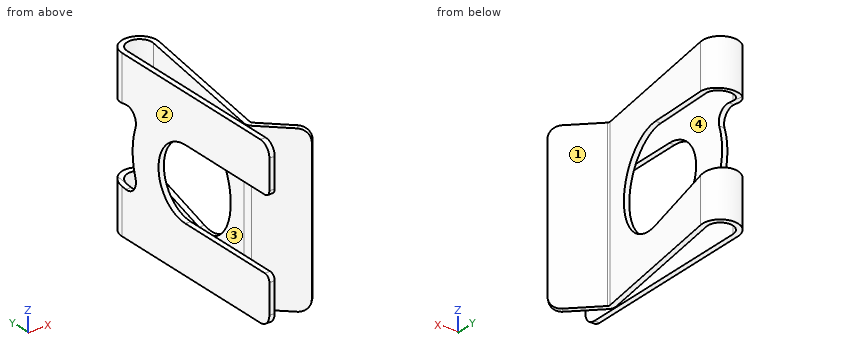
```python
from build123d import *

# Parameters (mm, degrees)
BOSS_EXTRUDE1_DEPTH      = 7
BOSS_EXTRUDE1_DEPTH_BACK = 7
CUT_EXTRUDE1_DEPTH       = 0.45
CUT_EXTRUDE2_DEPTH       = 3.9
CUT_EXTRUDE3_DEPTH       = 3.9
CUT_EXTRUDE4_DEPTH       = 0.45
CUT_EXTRUDE5_DEPTH       = 0.45
CUT_EXTRUDE6_DEPTH       = 0.45
CUT_EXTRUDE7_DEPTH       = 0.45
CUT_EXTRUDE8_DEPTH       = 0.9
CUT_EXTRUDE8_DEPTH_BACK  = 0.9


with BuildPart() as part:
    # Sketch1 → Boss-Extrude1 (new body, two sides)
    with BuildSketch(Plane.XY) as boss_extrude1_sk:
        with BuildLine():
            Line((0, 7.1), (0, -9.4))
            Line((0, -9.4), (0.45, -9.4))
            Line((0.45, -9.4), (0.45, 7.1))
            ThreePointArc((0.45, 7.1), (1.582064395, 8.146788152), (2.537172257, 6.936373264))
            Line((2.537172257, 6.936373264), (0.513952578, -5.888103783))
            ThreePointArc((0.513952578, -5.888103783), (0.540554577, -6.207374008), (0.711367038, -6.478416895))
            Line((0.711367038, -6.478416895), (3.64329211, -9.314940681))
            Line((3.64329211, -9.314940681), (3.956184866, -8.99152435))
            Line((3.956184866, -8.99152435), (1.024259794, -6.155000564))
            ThreePointArc((1.024259794, -6.155000564), (0.967322307, -6.064652935), (0.958454974, -5.958229527))
            Line((0.958454974, -5.958229527), (2.981674653, 6.86624752))
            ThreePointArc((2.981674653, 6.86624752), (1.61723485, 8.595411646), (0, 7.1))
        make_face()
    extrude(amount=BOSS_EXTRUDE1_DEPTH)
    extrude(boss_extrude1_sk.sketch, amount=-BOSS_EXTRUDE1_DEPTH_BACK)

    # Sketch2 → Cut-Extrude1 (cut)
    with BuildSketch(Plane(origin=(0, 0, 0), x_dir=(0, 0, -1), z_dir=(1, 0, 0))):
        with BuildLine():
            Line((-3, 0), (-3, -9.4))
            Line((-3, -9.4), (3, -9.4))
            Line((3, -9.4), (3, 0))
            ThreePointArc((3, 0), (0, 3), (-3, 0))
        make_face()
    extrude(amount=CUT_EXTRUDE1_DEPTH, mode=Mode.SUBTRACT)

    # Sketch3 → Cut-Extrude2 (cut)
    with BuildSketch(Plane(origin=(0.45, 0, 0), x_dir=(0, 0, -1), z_dir=(1, 0, 0))):
        with BuildLine():
            Line((3.97169805, 0.474989052), (3, 8.6))
            Line((3, 8.6), (-3, 8.6))
            Line((-3, 8.6), (-3.97169805, 0.474989052))
            ThreePointArc((-3.97169805, 0.474989052), (0, -4), (3.97169805, 0.474989052))
        make_face()
    extrude(amount=CUT_EXTRUDE2_DEPTH, mode=Mode.SUBTRACT)

    # Sketch4 → Cut-Extrude3 (cut)
    with BuildSketch(Plane(origin=(0.45, 0, 0), x_dir=(0, 0, -1), z_dir=(1, 0, 0))):
        with BuildLine():
            Line((3.233838828, 6.644718687), (3, 8.6))
            Line((3, 8.6), (-3, 8.6))
            Line((-3, 8.6), (-3.233838828, 6.644718687))
            ThreePointArc((-3.233838828, 6.644718687), (-2.869340143, 5.748101911), (-1.916144125, 5.580178464))
            ThreePointArc((-1.916144125, 5.580178464), (0, 5.9), (1.916144125, 5.580178464))
            ThreePointArc((1.916144125, 5.580178464), (2.869340143, 5.748101911), (3.233838828, 6.644718687))
        make_face()
    extrude(amount=-CUT_EXTRUDE3_DEPTH, mode=Mode.SUBTRACT)

    # Sketch5 → Cut-Extrude4 (cut)
    with BuildSketch(Plane(origin=(0, 0, 0), x_dir=(0, 0, -1), z_dir=(1, 0, 0))):
        with BuildLine():
            Line((-7, -9.4), (-6, -9.4))
            ThreePointArc((-6, -9.4), (-6.707106781, -9.107106781), (-7, -8.4))
            Line((-7, -8.4), (-7, -9.4))
        make_face()
    extrude(amount=CUT_EXTRUDE4_DEPTH, mode=Mode.SUBTRACT)

    # Sketch6 → Cut-Extrude5 (cut)
    with BuildSketch(Plane(origin=(0, 0, 0), x_dir=(0, 0, -1), z_dir=(1, 0, 0))):
        with BuildLine():
            Line((6, -9.4), (7, -9.4))
            Line((7, -9.4), (7, -8.4))
            ThreePointArc((7, -8.4), (6.707106781, -9.107106781), (6, -9.4))
        make_face()
    extrude(amount=CUT_EXTRUDE5_DEPTH, mode=Mode.SUBTRACT)

    # Sketch7 → Cut-Extrude6 (cut)
    with BuildSketch(Plane(origin=(0, 0, 0), x_dir=(0, 0, -1), z_dir=(1, 0, 0))):
        with BuildLine():
            Line((3, -9.4), (3.5, -9.4))
            ThreePointArc((3.5, -9.4), (3.146446609, -9.253553391), (3, -8.9))
            Line((3, -8.9), (3, -9.4))
        make_face()
    extrude(amount=CUT_EXTRUDE6_DEPTH, mode=Mode.SUBTRACT)

    # Sketch8 → Cut-Extrude7 (cut)
    with BuildSketch(Plane(origin=(0, 0, 0), x_dir=(0, 0, -1), z_dir=(1, 0, 0))):
        with BuildLine():
            Line((-3.5, -9.4), (-3, -9.4))
            Line((-3, -9.4), (-3, -8.9))
            ThreePointArc((-3, -8.9), (-3.146446609, -9.253553391), (-3.5, -9.4))
        make_face()
    extrude(amount=CUT_EXTRUDE7_DEPTH, mode=Mode.SUBTRACT)

    # Sketch9 → Cut-Extrude8 (cut, two sides)
    with BuildSketch(Plane(origin=(-2.580622377, -2.667416888, 0), x_dir=(0.718702958, -0.695317235, 0), z_dir=(0.695317235, 0.718702958, 0))) as cut_extrude8_sk:
        with BuildLine():
            Line((8.094816521, -7), (8.094816521, -8))
            Line((8.094816521, -8), (10.094816521, -8))
            Line((10.094816521, -8), (10.094816521, 8))
            Line((10.094816521, 8), (8.094816521, 8))
            Line((8.094816521, 8), (8.094816521, 7))
            ThreePointArc((8.094816521, 7), (8.801923302, 6.707106781), (9.094816521, 6))
            Line((9.094816521, 6), (9.094816521, -6))
            ThreePointArc((9.094816521, -6), (8.801923302, -6.707106781), (8.094816521, -7))
        make_face()
    extrude(amount=CUT_EXTRUDE8_DEPTH, mode=Mode.SUBTRACT)
    extrude(cut_extrude8_sk.sketch, amount=-CUT_EXTRUDE8_DEPTH_BACK, mode=Mode.SUBTRACT)


solid = part.part
```
Could you check a few things on this model? Use its own coordinates, in mm. Face numbers are marked on the shaded views. A direction names the side the tool comes from. Coordinates: 2 decimals unless noted, no trailing zeros. Order: outer loops, then holes, each group sorted by start corner. A loop starts at its lowest first (then second) coordinate and runs counter-clockwise, first axis right, second up. Notation, with made-up numbers: M 80.25,82 L 106.25,82 A22 cw 106.25,109 Z; hole C 53,53.5 d1. An arc over 180 degrees is marked long. Use a Markdown table: item, result. Add a question column.
Q1. I'm going to push a flat-ended pin straight in: pin 1 (3 mm diameter, centred on y = 2.5, z = -2.5, fed in from +X). Where does the tip first touch, or does it pass through?
Q2. I want a section at D-D on z = -5.25. List the corners of the cut face in (x, y) for me (3 decimals).
Q3. I want a section at B-B on y = 4.5. List the corners of the cut face in (x, z) for me.
Q4. Which directions (+Z, -Z, +X, -X, +Y, -Y) give clear straight access to the entire face, cutting with the end or side of a thin tool? Please do the marked faces 1, 2, 3 and 4.
Q5. If I drill on L1, parallel to Z at x = 1.6, y = 0; L2, parallel to X at y = 0.5, z = 4.75; L3, parallel to X at y = 3.75, z = -3, over which ranges is the centre line in solid material (lowest first)?
Q6. I want a section at A-A on z = -0.75. List the corners of the cut face in (x, y) for me (3 decimals), then the cut area to 3 significant figures.
Q7. I want a section at C-C on x = 1.3. List the corners of the cut face in (y, z) for me, then the cut area to 3 significant figures.
Checked values:
| question | item | result |
|---|---|---|
| 1 | pin 1 | x = 2.45 |
| 2 | outline | M 0,-9.4 L 0.45,-9.4 L 0.45,7.1 A1.05 cw long 2.537,6.936 L 0.514,-5.888 A0.675 ccw 0.711,-6.478 L 3.643,-9.315 L 3.956,-8.991 L 1.024,-6.155 A0.225 cw 0.958,-5.958 L 2.982,6.866 A1.5 ccw long 0,7.1 Z |
| 3 | outline | M 0,-7 L 0.45,-7 L 0.45,7 L 0,7 Z; M 2.15,-7 L 2.61,-7 L 2.61,-3.49 L 2.15,-3.49 Z; M 2.15,3.49 L 2.61,3.49 L 2.61,7 L 2.15,7 Z |
| 4 | face 1 | +Z, -Z, +X |
| 4 | face 2 | +Z, -Z, -X, +Y, -Y |
| 4 | face 3 | +Z, -Z |
| 4 | face 4 | +Z, -Z, -Y |
| 5 | L1 | -7 to -4, 4 to 7 |
| 5 | L2 | 0 to 0.45, 1.52 to 1.98 |
| 5 | L3 | 0 to 0.45 |
| 6 | outline | M 0,2.905 L 0.45,2.905 L 0.45,5.852 L 0,5.852 Z; M 0.514,-5.888 A0.675 ccw 0.711,-6.478 L 3.643,-9.315 L 3.956,-8.991 L 1.024,-6.155 A0.225 cw 0.958,-5.958 L 1.279,-3.929 L 0.823,-3.929 Z |
| 6 | area | 4.26 mm² |
| 7 | outline | M -7.05,-7 L -6.42,-7 L -6.42,7 L -7.05,7 Z; M -3.79,-7 L -0.91,-7 L -0.91,-3.9 A4 cw -3.79,-1.27 Z; M -3.79,1.27 A4 cw -0.91,3.9 L -0.91,7 L -3.79,7 Z; M 8.13,-7 L 8.59,-7 L 8.59,-3 L 8.13,-3.06 Z; M 8.13,3.06 L 8.59,3 L 8.59,7 L 8.13,7 Z |
| 7 | area | 35.2 mm² |
